Can you work these out from the model? Positions are in its coordinate system, mm. Face numbers are marked on the shaded views. A direction names the side the tool comes from. Give positions to 0.01 mm unless a question says otherwise; leave off trailing zeros. Order: outer loops, then holes, each group sorted by start corner. A loop starts at its lowest first (then second) coordinate and runs counter-clockwise, first axis right, second up. Notation, with made-up numbers: M 69,13.5 L 119,13.5 A11 cw 119,29.5 Z; hole C 57.25,-12 d11. An arc over 180 degrees is marked long. Answer as a JSON object with one key per item and string values.
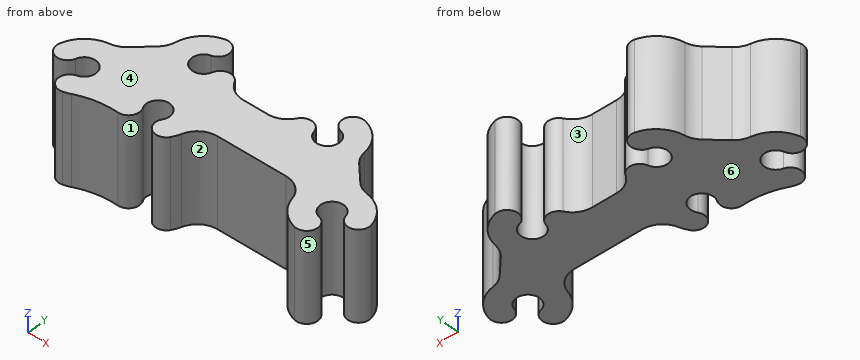
```python
from build123d import *

# Parameters (mm, degrees)
EXTRUDE1_DEPTH = 12.7


with BuildPart() as part:
    # Sketch1 → Extrude1 (new body, symmetric)
    with BuildSketch(Plane.XY):
        with BuildLine():
            Line((3.541744722, 6.350000317), (-3.541744722, 6.350000317))
            ThreePointArc((-3.541744722, 6.350000317), (-6.717339471, 7.201082424), (-9.041692685, 9.526189926))
            ThreePointArc((-9.041692685, 9.526189926), (-12.168838665, 11.052363462), (-14.755482048, 8.724806019))
            ThreePointArc((-14.755482048, 8.724806019), (-20.272604103, 7.166406874), (-18.823535008, 12.713247635))
            ThreePointArc((-18.823535008, 12.713247635), (-16.4863366, 16.468880196), (-20.266433142, 18.766301026))
            ThreePointArc((-20.266433142, 18.766301026), (-25.058481671, 15.875940516), (-27.400098665, 10.793151634))
            ThreePointArc((-27.400098665, 10.793151634), (-28.012836895, 8.894644494), (-29.184374008, 7.27993762))
            Line((-29.184374008, 7.27993762), (-33.668197009, 2.789809368))
            ThreePointArc((-33.668197009, 2.789809368), (-35.320246571, 1.597881998), (-37.264713426, 0.990422317))
            ThreePointArc((-37.264713426, 0.990422317), (-42.296938103, -1.364178798), (-45.159399664, -6.125874443))
            ThreePointArc((-45.159399664, -6.125874443), (-42.896712959, -9.899879208), (-39.1227081, -7.637192526))
            ThreePointArc((-39.1227081, -7.637192526), (-33.584022437, -6.104926504), (-35.119498005, -11.642723169))
            ThreePointArc((-35.119498005, -11.642723169), (-37.384371438, -15.415416021), (-33.611678586, -17.680289454))
            ThreePointArc((-33.611678586, -17.680289454), (-32.609025986, -17.370294909), (-31.646563329, -16.951875875))
            ThreePointArc((-31.646563329, -16.951875875), (-26.066681379, -15.174096844), (-20.21993522, -14.840719891))
            ThreePointArc((-20.21993522, -14.840719891), (-17.353189866, -13.362481197), (-17.337180754, -10.137087846))
            ThreePointArc((-17.337180754, -10.137087846), (-14.434495922, -5.136768789), (-11.74460461, -10.254703395))
            ThreePointArc((-11.74460461, -10.254703395), (-10.54959622, -14.439704472), (-6.339625545, -13.335881127))
            ThreePointArc((-6.339625545, -13.335881127), (-5.758478435, -12.199696418), (-5.334434584, -10.996021018))
            ThreePointArc((-5.334434584, -10.996021018), (-3.058049309, -7.643184473), (0.782668949, -6.35))
            Line((0.782668949, -6.35), (20.629531136, -6.35))
            ThreePointArc((20.629531136, -6.35), (24.469498585, -7.642614313), (26.746128433, -10.994204727))
            ThreePointArc((26.746128433, -10.994204727), (29.278173872, -15.26179643), (33.613137194, -17.676684799))
            ThreePointArc((33.613137194, -17.676684799), (37.385829768, -15.411811583), (35.120956636, -11.639118675))
            ThreePointArc((35.120956636, -11.639118675), (33.586157492, -6.100645238), (39.124630957, -7.635444299))
            ThreePointArc((39.124630957, -7.635444299), (42.897323989, -9.900317715), (45.162197311, -6.127624707))
            ThreePointArc((45.162197311, -6.127624707), (42.301720517, -1.363571666), (37.269569316, 0.993541642))
            ThreePointArc((37.269569316, 0.993541642), (35.33100147, 1.598861028), (33.682682253, 2.785242337))
            Line((33.682682253, 2.785242337), (29.191501523, 7.268011131))
            ThreePointArc((29.191501523, 7.268011131), (27.998435311, 8.921281589), (27.390796294, 10.867427785))
            ThreePointArc((27.390796294, 10.867427785), (25.0373104, 15.90083737), (20.275755297, 18.764698607))
            ThreePointArc((20.275755297, 18.764698607), (16.501386803, 16.503215052), (18.762343911, 12.728531392))
            ThreePointArc((18.762343911, 12.728531392), (20.292630817, 7.189814806), (14.755356019, 8.725310571))
            ThreePointArc((14.755356019, 8.725310571), (12.168581157, 11.052399567), (9.041692685, 9.526189926))
            ThreePointArc((9.041692685, 9.526189926), (6.717339471, 7.201082424), (3.541744722, 6.350000317))
        make_face()
    extrude(amount=EXTRUDE1_DEPTH, both=True)


solid = part.part
```
1) Thinking about a two-plate mould opening in Z: for the marked faces 4, 5 and 6, which applies, pulls with the +Z half, pulls with the -Z half, needs draft (parallel to the pull), parting line crosses it, or undercut?
Results found:
{"face 4": "pulls with the +Z half", "face 5": "needs draft", "face 6": "pulls with the -Z half"}
2) For the marked faces 1, 2 and 3, which set-ups out of +Z, -Z, +X, -X, +Y, -Y let a thin tool reach every point of the face, with its end or its side?
Results found:
{"face 1": "+Z, -Z", "face 2": "+Z, -Z, -Y", "face 3": "+Z, -Z, +Y"}
3) I want a section at B-B on x = 24.5. Write out the boundary of the cut face in (y, z), and give its area (3 significant figures).
Results found:
{"outline": "M -7.67,-12.7 L 16.45,-12.7 L 16.45,12.7 L -7.67,12.7 Z", "area": "613 mm²"}
4) I'm going to push flat-ended pins straight in: pin 1 Ø1 at (y, z) = (10.5, 8) entering from +X; pin 2 Ø8 at (x, z) = (1.5, 5) entering from +Y; pin 3 Ø2 at (x, z) = (27, 0.5) entering from +Y. Where does each tip first touch, or does it pass through?
Results found:
{"pin 1": "stops at x = 27.58", "pin 2": "stops at y = 6.66", "pin 3": "stops at y = 14.63"}
5) I need wall thicknesses on L1, parallel to X at y = -8, z = 9.5; L2, parallel to Y at x = 1, z = -4.75; L3, parallel to Y at x = -36, z = -3.75. Which ranges of each line are inside material? Lowest first, please.
Results found:
{"L1": "x = -45.04 to -39.24, -32.65 to -17.78, -11.23 to -3.49, 24.9 to 32.65, 39.24 to 45.05", "L2": "y = -6.35 to 6.35", "L3": "y = -17.31 to -12.01, -5.14 to 1.31"}
6) I want a section at A-A on y = 5. Write out the boundary of the cut face in (x, z), and give its area (3 significant figures).
Results found:
{"outline": "M -31.46,-12.7 L 31.46,-12.7 L 31.46,12.7 L -31.46,12.7 Z", "area": "1,600 mm²"}
